Build history of the part. All positions in model axes, mm. A direction names the side the tool comes from. Give positions to 0.01 mm unless a question says otherwise; leave off trailing zeros. Order: outer loops, then holes, each group sorted by start corner. A loop starts at its lowest first (then second) coordinate and runs counter-clockwise, first axis right, second up. Notation, with made-up numbers: (-11.5, 77.5) -> (14.5, 77.5) arc R21 ccw to (14.5, 112.5) -> close; hole circle Ø10 at (24, -18). An arc over 180 degrees is marked (long way). Use a Markdown table: item, result. Add a question column.
```python
from build123d import *

# Parameters (mm, degrees)
BOSS_EXTRUDE1_DEPTH         = 10.4
BOSS_EXTRUDE2_DEPTH         = 15
TAP_DRILL_FOR_M3_TAP1_D     = 2.5
TAP_DRILL_FOR_M3_TAP1_DEPTH = 3
TAP_DRILL_FOR_M3_TAP1_TIP   = 0.751075774


with BuildPart() as part:
    # Sketch1 → Boss-Extrude1 (new, symmetric)
    with BuildSketch(Plane.XY):
        Polygon((-10, 0), (-5, 0), (-5, -0.3), (5, -0.3), (5, 0), (10, 0), (10, -8), (4.5, -8), (4.5, -4), (-4.5, -4), (-4.5, -8), (-10, -8), align=None)
    extrude(amount=BOSS_EXTRUDE1_DEPTH, both=True)

    # Sketch2 → Boss-Extrude2 (add, symmetric)
    with BuildSketch(Plane.XY):
        Polygon((-9.65, -0.8), (9.65, -0.8), (9.65, -8), (4.5, -8), (4.5, -4), (-4.5, -4), (-4.5, -8), (-9.65, -8), align=None)
    extrude(amount=BOSS_EXTRUDE2_DEPTH, both=True)

    # Tap Drill for M3 Tap1
    with Locations(Plane(origin=(0, 0, 0), x_dir=(1, 0, 0), z_dir=(0, 1, 0))):
        with Locations((7.5, 5), (7.5, -5), (-7.5, 5), (-7.5, -5)):
            Hole(TAP_DRILL_FOR_M3_TAP1_D / 2, depth=TAP_DRILL_FOR_M3_TAP1_DEPTH)
            with Locations((0, 0, -(TAP_DRILL_FOR_M3_TAP1_DEPTH + TAP_DRILL_FOR_M3_TAP1_TIP / 2))):  # 118° drill point
                Cone(0, TAP_DRILL_FOR_M3_TAP1_D / 2, TAP_DRILL_FOR_M3_TAP1_TIP, mode=Mode.SUBTRACT)


solid = part.part
```
(1) Wall check: probe 1 along X at (y, z) = (-1.6, 5); probe 2 along Z at (x, y) = (-7.5, -1.5); probe 3 along X at (y, z) = (-6, 1.75). Give the ranges that are in metal, low to high.
(2) Tool access for faces 1 (the face through (-9.65, -4, -13)), 2 (the face through (9.65, -4, 13)), 3 (the face through (4.5, -6, 0)), 4 (the face through (9.65, -4, -13)), 5 (the face through (8.49, -1.52, 5.76)): list every direction of +Z, -Z, +X, -X, +Y, -Y with a clear straight run to the whole face (end or side of a thin tool).
(3) Band-saw the part on A-A on y = -5. Give the cut face in (x, z).
(4) Pin check, flat tips, straight feed: pin 1 Ø2 at (x, z) = (-7.5, -5) entering from +Y; pin 2 Ø2 at (x, z) = (3, -1) entering from +Y; pin 3 Ø1.5 at (x, z) = (1.5, -3.5) entering from -Y. Stop position of each tip, or through.
(5) Band-saw the part on B-B on z = -9.5. Give the cut face in (x, y), plus the area to 3 significant figures.
(6) Mould opens along Z. For faces 6 (the face through (-10, -4, 0)), 7 (the face through (7.34, -3.62, -5.15)) say: released by +Z, released by -Z, zero draft, split by the parting line, or undercut.
Response:
| question | item | result |
|---|---|---|
| 1 | probe 1 | x = -10 to -8.75, -6.25 to 6.25, 8.75 to 10 |
| 1 | probe 2 | z = -15 to -6.25, -3.75 to 3.75, 6.25 to 15 |
| 1 | probe 3 | x = -10 to -4.5, 4.5 to 10 |
| 2 | face 1 | -Z, -X, +Y, -Y |
| 2 | face 2 | +Z, +X, +Y, -Y |
| 2 | face 3 | +Z, -Z, -Y |
| 2 | face 4 | -Z, +X, +Y, -Y |
| 2 | face 5 | +Y |
| 3 | outline | (-10, -10.4) -> (-9.65, -10.4) -> (-9.65, -15) -> (-4.5, -15) -> (-4.5, 15) -> (-9.65, 15) -> (-9.65, 10.4) -> (-10, 10.4) -> close; (4.5, -15) -> (9.65, -15) -> (9.65, -10.4) -> (10, -10.4) -> (10, 10.4) -> (9.65, 10.4) -> (9.65, 15) -> (4.5, 15) -> close |
| 4 | pin 1 | stops at y = -3.15 |
| 4 | pin 2 | stops at y = -0.3 |
| 4 | pin 3 | stops at y = -4 |
| 5 | outline | (-10, -8) -> (-4.5, -8) -> (-4.5, -4) -> (4.5, -4) -> (4.5, -8) -> (10, -8) -> (10, 0) -> (5, 0) -> (5, -0.3) -> (-5, -0.3) -> (-5, 0) -> (-10, 0) -> close |
| 5 | area | 121 mm² |
| 6 | face 6 | zero draft |
| 6 | face 7 | undercut |
